CAD build for the part. Positions are in the model's coordinates, mm. Round coordinates to 2 decimals unless told otherwise and drop trailing zeros. Loops run counter-clockwise (first coordinate to the right, second up) from the corner with the lowest first, then second, coordinate; pieces in that order, holes last. Notation, with made-up numbers: M 18,22.25 L 39,22.25 A26 ccw 39,52.25 Z; hole C 57.25,-30.75 d6. An arc over 180 degrees is marked long. Use a Markdown table: item, result. Add a question column.
(1) Band-saw the part on B-B, the plane x = 62. Write the cut outline in (y, z), and give its area (3 significant figures).
(2) Two-plate mould, pull along Y, no slides. Class faces 1 (the face through (248, -198, 10)), 2 (the face through (-336.674, -14.817, 4.93)), 3 (the face through (-41.3, -314.3, 4.9)): released by +Y, released by -Y, zero draft, split by the parting line, or undercut.
(3) Wall check: L1, parallel to Y at x = 0, z = 5.5; L2, parallel to X at y = -279, z = 5; L3, parallel to Y at x = -163.5, z = 2.5. Give the ranges that are in metal, low to high.
(4) Flat gauge pins, fed straight in: P1, Ø11, axis at x = 283.19, y = 163.5, coming from the +Z side; P2, Ø4, axis at x = 30, z = 3, coming from the +Y side; P3, Ø4, axis at y = -160.5, z = 3, coming from the +X side; P4, Ø4, axis at x = 205, z = 5.5, coming from the -Y side. Where does each tip first touch, or does it go through?
(5) Band-saw the part on C-C, the plane z = 1.5. Give the number of separate pieces and of enclosed holes in the cut face, and give its area (3 significant figures).
(6) Band-saw the part on A-A, the plane y = 65. Write the cut outline in (x, z), and give its area (3 significant figures).
Autodesk Inventor part; units mm, degrees
ref_plane "YZ Plane" through (0, 0, 0) normal (1, 0, 0) x (0, 1, 0)
ref_plane "XZ Plane" through (0, 0, 0) normal (0, 1, 0) x (-1, 0, 0)
ref_plane "XY Plane" through (0, 0, 0) normal (0, 0, 1) x (1, 0, 0)
sketch "Boceto1" plane through (0, 0, 0) normal (0, 0, 1) x (1, 0, 0)
  circle A0 centre (0, 0) radius 337
  circle A1 centre (0, 0) radius 317
  dimension "d0" = 674
  dimension "d1" = 634
extrude "Extrusión1" add sketch "Boceto1" along normal blind 10
sketch "Boceto2" plane through (0, 0, 10) normal (0, 0, 1) x (1, 0, 0)
  circle A0 centre (0, 0) radius 327 construction
  circle A1 centre (0, 0) radius 337
  circle A2 centre (0, 327) radius 6.75
  circle A3 centre (-163.5, 283.1903) radius 6.75
  circle A4 centre (-283.1903, 163.5) radius 6.75
  circle A5 centre (-327, 0) radius 6.75
  circle A6 centre (-283.1903, -163.5) radius 6.75
  circle A7 centre (-163.5, -283.1903) radius 6.75
  circle A8 centre (0, -327) radius 6.75
  circle A9 centre (163.5, -283.1903) radius 6.75
  circle A10 centre (283.1903, -163.5) radius 6.75
  circle A11 centre (327, 0) radius 6.75
  circle A12 centre (283.1903, 163.5) radius 6.75
  circle A13 centre (163.5, 283.1903) radius 6.75
  dimension "d4" = 10
  dimension "d5" = 13.5
  dimension "d8" = 360
extrude "Extrusión2" cut sketch "Boceto2" against normal through all contours A2 | A3 | A4 | A5 | A6 | A7 | A8 | A9 | A10 | A11 | A12 | A13
properties part number "Aro del tambor"
Return value:
| question | item | result |
|---|---|---|
| 1 | outline | M -331.25,0 L -310.88,0 L -310.88,10 L -331.25,10 Z; M 310.88,0 L 331.25,0 L 331.25,10 L 310.88,10 Z |
| 1 | area | 407 mm^2 |
| 2 | face 1 | zero draft |
| 2 | face 2 | split by the parting line |
| 2 | face 3 | undercut |
| 3 | L1 | -337 to -333.75, -320.25 to -317, 317 to 320.25, 333.75 to 337 |
| 3 | L2 | -189.02 to -168.79, -158.21 to -150.49, 150.49 to 158.21, 168.79 to 189.02 |
| 3 | L3 | -294.68 to -289.94, -276.44 to -271.58, 271.58 to 276.44, 289.94 to 294.68 |
| 4 | P1 | through |
| 4 | P2 | y = 335.83 |
| 4 | P3 | x = 297.4 |
| 4 | P4 | y = -269 |
| 5 | separate pieces | 1 |
| 5 | enclosed holes | 13 |
| 5 | area | 39,400 mm^2 |
| 6 | outline | M -330.67,0 L -310.26,0 L -310.26,10 L -330.67,10 Z; M 310.26,0 L 330.67,0 L 330.67,10 L 310.26,10 Z |
| 6 | area | 408 mm^2 |
